Verification items for the finished model (mm, model axes). A direction names the side the tool comes from. Round coordinates to 2 decimals unless told otherwise and drop trailing zeros. Order: outer loops, then holes, each group sorted by start corner. A loop starts at its lowest first (then second) coordinate and runs counter-clockwise, first axis right, second up. Notation, with made-up numbers: (14, 84) -> (19, 84) arc R23 cw to (19, 117) -> close; hole circle Ø11 at (-20.5, 51). An arc over 180 degrees is marked (long way). Return JSON: item names as keys, results as strings. Group by question number.
Item 1: Sectioned sample at B-B on x = -11.5. Record the cut outline in (y, z), plus the area to 3 significant figures.
Item 2: Sectioned sample at C-C on z = 0.9. Give the number of separate pieces and of enclosed holes in the cut face, plus the area to 3 significant figures.
Item 3: Access from +Z, -Z, +X, -X, +Y, -Y to the whole of each face (thin tool, end or side, straight path). Record for faces 1 (the flat face through (-11, 20, 1)), 2 (the flat face through (0, 8.1, 2)), 3 (the flat face through (11, -20, 1)), 4 (the flat face through (27.5, 21, 1)), 5 (the flat face through (-44, 20, 1)).
Item 4: Sectioned sample at A-A on y = 0. Record the cut outline in (x, z), plus the area to 3 significant figures.
Item 5: Depth check by flat-ended pin: pin 1 Ø4 at (x, y) = (20, 7.5) entering from -Z; pin 2 Ø1.5 at (x, z) = (-10.5, 1) entering from +Y; pin 3 Ø1.5 at (y, z) = (-22, 1) entering from +X; pin 4 Ø1 at (x, z) = (-10, 0.5) entering from -Y. Enter the tip coordinate at first touch or a pass-through.
Item 6: Sectioned sample at D-D on x = -40. Record the cut outline in (y, z), plus the area to 3 significant figures.
Item 7: Draft check along Y on faces 6 (the flat face through (-27.5, 21, 1)), 7 (the cylindrical face through (-21.1, 7.5, 1.5)), 8 (the flat face through (22, -23, 1)). Enter one of: pulls with the +Y half, pulls with the -Y half, needs draft (parallel to the pull), parting line crosses it, or undercut.
Item 8: Scan lines: probe 1 along X at (y, z) = (-20.5, 2.3); probe 2 along Y at (x, z) = (-20, 2.05); probe 3 along Y at (x, z) = (20, 0.75). Record each from-to range of solid material in increasing order. Write a range as from..to.
```python
from build123d import *

# Parameters (mm, degrees)
SKETCH1_W           = 10
SKETCH1_H           = 3
BOSS_EXTRUDE1_DEPTH = 3
SKETCH2_R           = 1.1
SKETCH2_R_2         = 1.25
SKETCH2_R_3         = 8.1
CUT_EXTRUDE1_DEPTH  = 65.327288144
SKETCH3_W           = 25.4
SKETCH3_H           = 16.2
CUT_EXTRUDE2_DEPTH  = 65.327288144


with BuildPart() as part:
    # Sketch1 → Boss-Extrude1 (new body)
    with BuildSketch(Plane.XY):
        Polygon((-60, 20), (-60, 0), (60, 0), (60, 20), (27.5, 20), (17.5, 20), (5, 20), (-5, 20), (-17.5, 20), (-27.5, 20), align=None)
        Polygon((60, 0), (-60, 0), (-60, -20), (-27.5, -20), (-17.5, -20), (-5, -20), (5, -20), (17.5, -20), (27.5, -20), (60, -20), align=None)
        with Locations((-22.5, 21.5)):
            Rectangle(SKETCH1_W, SKETCH1_H)
        with Locations((0, 21.5)):
            Rectangle(SKETCH1_W, SKETCH1_H)
        with Locations((22.5, 21.5)):
            Rectangle(SKETCH1_W, SKETCH1_H)
        with Locations((22.5, -21.5)):
            Rectangle(SKETCH1_W, SKETCH1_H)
        with Locations((0, -21.5)):
            Rectangle(SKETCH1_W, SKETCH1_H)
        with Locations((-22.5, -21.5)):
            Rectangle(SKETCH1_W, SKETCH1_H)
    extrude(amount=BOSS_EXTRUDE1_DEPTH)

    # Sketch2 → Cut-Extrude1 (cut, through all)
    with BuildSketch(Plane.XY.offset(3)):
        with Locations((-20, 7.5)):
            Circle(SKETCH2_R)
        with Locations(Location((-20, -7.5, 0), (0, 0, 180))):
            Circle(SKETCH2_R_2)
        with Locations((20, -7.5)):
            Circle(SKETCH2_R_2)
        with Locations(Location((20, 7.5, 0), (0, 0, 180))):
            Circle(SKETCH2_R_2)
        with Locations((-12.7, 0)):
            Circle(SKETCH2_R_3)
        with Locations((12.7, 0)):
            Circle(SKETCH2_R_3)
    extrude(amount=-CUT_EXTRUDE1_DEPTH, mode=Mode.SUBTRACT)

    # Sketch3 → Cut-Extrude2 (cut, through all)
    with BuildSketch(Plane.XY.offset(3)):
        Rectangle(SKETCH3_W, SKETCH3_H)
    extrude(amount=-CUT_EXTRUDE2_DEPTH, mode=Mode.SUBTRACT)


solid = part.part
```
Recorded:
{
 "1": {"outline": "(-20, 0) -> (-8.1, 0) -> (-8.1, 3) -> (-20, 3) -> close; (8.1, 0) -> (20, 0) -> (20, 3) -> (8.1, 3) -> close", "area": "71.4 mm²"},
 "2": {"separate pieces": "1", "enclosed holes": "5", "area": "4,340 mm²"},
 "3": {"face 1": "+Z, -Z, +Y", "face 2": "+Z, -Z", "face 3": "+Z, -Z, -Y", "face 4": "+Z, -Z, +X, +Y", "face 5": "+Z, -Z, -X, +Y"},
 "4": {"outline": "(-60, 0) -> (-20.8, 0) -> (-20.8, 3) -> (-60, 3) -> close; (20.8, 0) -> (60, 0) -> (60, 3) -> (20.8, 3) -> close", "area": "235 mm²"},
 "5": {"pin 1": "z = 0", "pin 2": "y = 20", "pin 3": "x = 27.5", "pin 4": "y = -20"},
 "6": {"outline": "(-20, 0) -> (20, 0) -> (20, 3) -> (-20, 3) -> close", "area": "120 mm²"},
 "7": {"face 6": "needs draft", "face 7": "undercut", "face 8": "pulls with the -Y half"},
 "8": {"probe 1": "-27.5..-17.5, -5..5, 17.5..27.5", "probe 2": "-23..-8.75, -6.25..-3.51, 3.51..6.4, 8.6..23", "probe 3": "-23..-8.75, -6.25..-3.51, 3.51..6.25, 8.75..23"}
}
